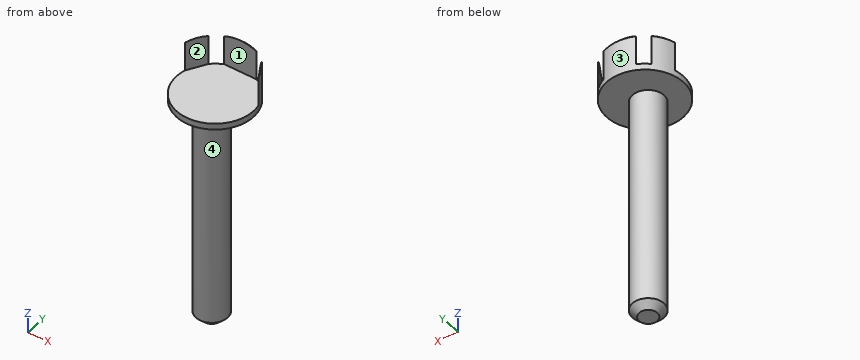
```python
from build123d import *

# Parameters (mm, degrees)
SKETCH1_R          = 1.778
EXTRUDE1_DEPTH     = 25.4
SKETCH3_R          = 4.318
EXTRUDE3_DEPTH     = 4.7625
CHAMFER1_SIZE      = 0.762
CUT_EXTRUDE1_DEPTH = 4.064


with BuildPart() as part:
    # Sketch1 → Extrude1 (new body)
    with BuildSketch(Plane.XY):
        Circle(SKETCH1_R)
    extrude(amount=EXTRUDE1_DEPTH)

    # Sketch3 → Extrude3 (add)
    with BuildSketch(Plane.XY.offset(25.4)):
        with Locations(Location((0, 0.491553118, 0), (0, 0, 180))):
            Circle(SKETCH3_R)
    extrude(amount=EXTRUDE3_DEPTH)

    # Chamfer1
    chamfer1_edges = [part.edges().sort_by_distance(p)[0] for p in [
        (-1.778, 0, 0),
        (4.318, 0.491553118, 30.1625),
    ]]
    chamfer(chamfer1_edges, length=CHAMFER1_SIZE)

    # Sketch4 → Cut-Extrude1 (cut)
    with BuildSketch(Plane.XY.offset(30.1625)):
        Polygon((5.08, 0), (2.54, 4.399409051), (-2.54, 4.399409051), (-5.08, 0), (-2.54, -4.399409051), (2.54, -4.399409051), align=None)
    extrude(amount=-CUT_EXTRUDE1_DEPTH, mode=Mode.SUBTRACT)


solid = part.part
```
The model under review builds one solid part; all positions refer to its coordinate system, in mm. Face numbers are marked on the shaded views. A direction names the side the tool comes from. Give positions to 0.01 mm unless a question says otherwise; leave off trailing zeros. Write each loop counter-clockwise with the first axis right and the second up, starting at its lowest first coordinate (ties: lowest second). Pieces come first, ordered by that corner, then holes. Notation, with made-up numbers: (-4, -36.5) -> (2, -36.5) arc R12 ccw to (2, -23.5) -> close; hole circle Ø7 at (-39, -33.75). An arc over 180 degrees is marked (long way). Put each result on its own line as item: value.
(1) We need section C-C, the plane y = 0. Give the boundary of the cut face in (x, z), and give its area (3 significant figures).
Results are:
outline: (-4.29, 25.4) -> (-1.78, 25.4) -> (-1.78, 0.76) -> (-1.02, 0) -> (1.02, 0) -> (1.78, 0.76) -> (1.78, 25.4) -> (4.29, 25.4) -> (4.29, 26.1) -> (-4.29, 26.1) -> close
area: 95.7 mm²
(2) For pin 1 Ø5 at (x, z) = (-0.5, 18) entering from +Y; pin 2 Ø2.5 at (x, y) = (2, 2) entering from -Z; pin 3 Ø1.5 at (x, y) = (0.5, 1) entering from +Z; pin 4 Ø1 at (y, z) = (-2.5, 7) entering from -X, all flat-tipped, find the tip position at first contact; note any pin that passes through.
Results are:
pin 1: y = 1.78
pin 2: z = 0.56
pin 3: z = 26.1
pin 4: through
(3) We need section B-B, the plane z = 4.5. Give the boundary of the cut face in (x, y), and give its area (3 significant figures).
Results are:
outline: circle Ø3.56 at (0, 0)
area: 9.93 mm²
(4) We need section D-D, the plane x = -2.25. Give the boundary of the cut face in (y, z), and give its area (3 significant figures).
Results are:
outline: (-3.19, 25.4) -> (4.18, 25.4) -> (4.18, 26.1) -> (-3.19, 26.1) -> close
area: 5.15 mm²
(5) Tool access review of the marked faces 1, 2, 3 and 4: name each direction out of +Z, -Z, +X, -X, +Y, -Y from which nothing blocks a thin tool from reaching the whole face with its end or side.
Results are:
face 1: +Z, +X, -X, -Y
face 2: +Z, -Y
face 3: +Z, -Z
face 4: -Z
(6) We need section A-A, the plane x = 0. Give the boundary of the cut face in (y, z).
Results are:
outline: (-3.83, 25.4) -> (-1.78, 25.4) -> (-1.78, 0.76) -> (-1.02, 0) -> (1.02, 0) -> (1.78, 0.76) -> (1.78, 25.4) -> (4.81, 25.4) -> (4.81, 29.4) -> (4.4, 29.81) -> (4.4, 26.1) -> (-3.83, 26.1) -> close
(7) To check wall thickness, follow probe 1 along Z at (x, y) = (-2.5, -0.5); probe 2 along X at (y, z) = (0.25, 26); probe 3 along Z at (x, y) = (-0.75, -0.25). State the ranges of each line that lie inside material, in increasing order. Write a range as from..to.
Results are:
probe 1: 25.4..26.1
probe 2: -4.31..4.31
probe 3: 0..26.1
